For this review, take the finished solid that the model builds, in its own axes (mm). Face numbers are marked on the shaded views. A direction names the side the tool comes from. Coordinates: 2 decimals unless noted, no trailing zeros. Loops run counter-clockwise (first coordinate to the right, second up) from the corner with the lowest first, then second, coordinate; pieces in that order, holes last. Notation, with made-up numbers: (-31.75, -21) - (-11.75, -21) arc R28 cw to (-11.75, 0) - close; hole circle Ø5 at (36, 67.5). An arc over 180 degrees is marked (long way). Answer as a JSON object with one key per item and string values. Group by question number.
Item 1: Tool access review of the marked faces 1 and 2: name each direction out of +Z, -Z, +X, -X, +Y, -Y from which nothing blocks a thin tool from reaching the whole face with its end or side.
Item 2: We need section A-A (x = -5.5). Give the boundary of the cut face in (y, z).
Item 3: We need section C-C (x = -42). Give the boundary of the cut face in (y, z).
Item 4: Mouldability with a two-part tool opening along Y and no side actions: class the marked faces 3, 4 and 5 as released by +Y, released by -Y, zero draft, split by the parting line, or undercut.
Item 5: To check wall thickness, follow line 1 (Y direction, x = -36, z = -2.75); line 2 (Y direction, x = -18.5, z = 0); line 3 (X direction, y = 1.5, z = 9). State the ranges of each line that lie inside material, in increasing order.
Item 6: We need section D-D (y = 1). Give the boundary of the cut face in (x, z).
Item 7: Clearance check with flat-ended pins moving along their axes: pin 1 (1.5 mm diameter, centred on x = -7.5, z = -4.5, fed in from +Y); pin 2 (6 mm diameter, centred on y = -5.5, z = 0.5, fed in from +X); pin 3 (17.5 mm diameter, centred on x = -3, y = 38, fed in from -Z); pin 4 (4 mm diameter, centred on x = 0, z = 1, fed in from -Y). State where each tip first meets the part, or that it passes through.
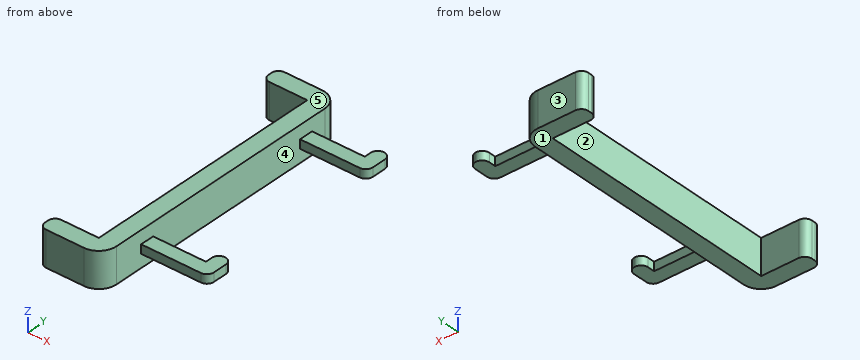
from build123d import *

# Parameters (mm, degrees)
BOSS_EXTRUDE1_DEPTH      = 10
BOSS_EXTRUDE1_DEPTH_BACK = 10
BOSS_EXTRUDE2_DEPTH      = 2.5
BOSS_EXTRUDE2_DEPTH_BACK = 2.5
FILLET1_R                = 10
FILLET2_R                = 4
FILLET3_R                = 4


with BuildPart() as part:
    # Sketch1 → Boss-Extrude1 (new, two sides: drawn at the far end of the back side and taken through both)
    with BuildSketch(Plane.XY.offset(-BOSS_EXTRUDE1_DEPTH_BACK)):
        Polygon((-22.510382525, 3.694889185), (-22.510382525, 30.211555852), (-22.510382525, 56.728222519), (-57.910382525, 56.728222519), (-57.910382525, 46.728222519), (-32.510382525, 46.728222519), (-32.510382525, -92.371777481), (-57.910382525, -92.371777481), (-57.910382525, -102.371777481), (-22.510382525, -102.371777481), (-22.510382525, -75.855110815), (-22.510382525, -49.338444148), (-22.510382525, -22.821777481), align=None)
    extrude(amount=BOSS_EXTRUDE1_DEPTH + BOSS_EXTRUDE1_DEPTH_BACK)

    # Sketch1<3> → Boss-Extrude2 (add, two sides: drawn at the far end of the back side and taken through both)
    with BuildSketch(Plane.XY.offset(-BOSS_EXTRUDE2_DEPTH_BACK)):
        Polygon((7.489617475, 38.211555852), (-22.510382525, 38.211555852), (-22.510382525, 30.211555852), (15.489617475, 30.211555852), (15.489617475, 46.211555852), (7.489617475, 46.211555852), align=None)
        Polygon((7.489617475, -67.855110815), (-22.510382525, -67.855110815), (-22.510382525, -75.855110815), (15.489617475, -75.855110815), (15.489617475, -59.855110815), (7.489617475, -59.855110815), align=None)
    extrude(amount=BOSS_EXTRUDE2_DEPTH + BOSS_EXTRUDE2_DEPTH_BACK)

    # Fillet1
    fillet1_edges = [part.edges().sort_by_distance(p)[0] for p in [
        (-22.510382525, -102.371777481, 0),
        (-22.510382525, 56.728222519, 0),
    ]]
    fillet(fillet1_edges, radius=FILLET1_R)

    # Fillet2
    fillet2_edges = [part.edges().sort_by_distance(p)[0] for p in [
        (-57.910382525, -102.371777481, 0),
        (-57.910382525, -92.371777481, 0),
        (7.489617475, -59.855110815, 0),
        (15.489617475, -59.855110815, 0),
        (15.489617475, -75.855110815, 0),
        (7.489617475, 46.211555852, 0),
        (15.489617475, 46.211555852, 0),
        (15.489617475, 30.211555852, 0),
        (-57.910382525, 56.728222519, 0),
    ]]
    fillet(fillet2_edges, radius=FILLET2_R - 0.0001)  # a hair under: the kernel refuses the full size

    # Fillet3
    fillet3_edges = [part.edges().sort_by_distance(p)[0] for p in [
        (-57.910382525, 46.728222519, 0),
    ]]
    fillet(fillet3_edges, radius=FILLET3_R)


solid = part.part
Check sheet entries:
{
 "1": {"face 1": "-Z, +X, -X, +Y, -Y", "face 2": "+Z, -Z, -X"},
 "2": {"outline": "(-75.86, -2.5) - (-67.86, -2.5) - (-67.86, 2.5) - (-75.86, 2.5) - close; (30.21, -2.5) - (38.21, -2.5) - (38.21, 2.5) - (30.21, 2.5) - close"},
 "3": {"outline": "(-102.37, -10) - (-92.37, -10) - (-92.37, 10) - (-102.37, 10) - close; (46.73, -10) - (56.73, -10) - (56.73, 10) - (46.73, 10) - close"},
 "4": {"face 3": "released by +Y", "face 4": "undercut", "face 5": "zero draft"},
 "5": {"line 1": "y = -102.37 to -92.37, 46.73 to 56.73", "line 2": "y = -75.86 to -67.86, 30.21 to 38.21", "line 3": "x = -32.51 to -22.51"},
 "6": {"outline": "(-32.51, -10) - (-22.51, -10) - (-22.51, 10) - (-32.51, 10) - close"},
 "7": {"pin 1": "passes through", "pin 2": "stops at x = -22.51", "pin 3": "stops at z = -2.5", "pin 4": "stops at y = -75.86"}
}
